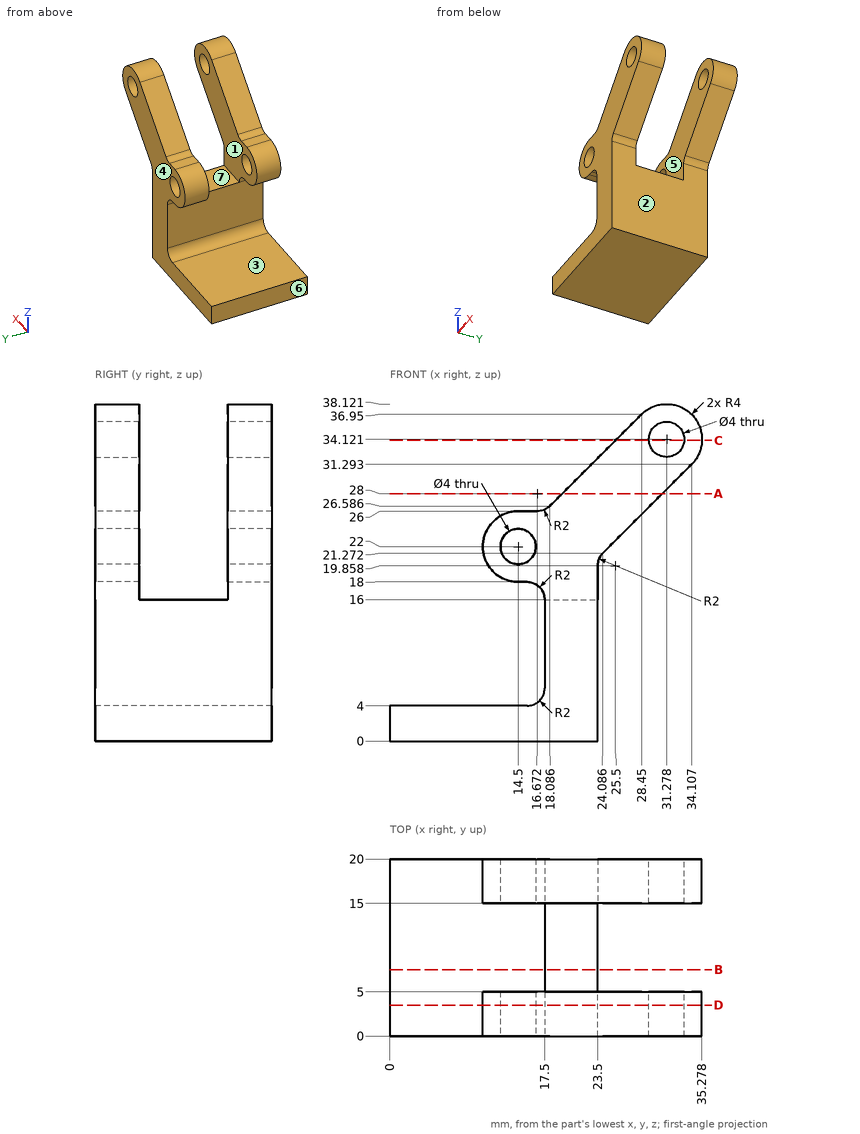
Could you check a few things on this drawing? It's one solid part, dimensions in mm from its lowest x, y, z. A direction names the side the tool comes from. Coordinates: 2 decimals unless noted, no trailing zeros. Order: outer loops, then holes, each group sorted by start corner. A loop starts at its lowest first (then second) coordinate and runs counter-clockwise, first axis right, second up. Notation, with made-up numbers: (61, 54.25) -> (112, 54.25) arc R28 ccw to (112, 90.25) -> close; hole circle Ø1 at (30, 28.25). An arc over 180 degrees is marked (long way). One line per item, written item: value. Start each with the question number.
1) We'd pull the mould along Y, two halves only. Please class the marked faces 4, 5, 6 and 7: +Y half, -Y half, draft (parallel to the pull), parting line (faces both ways), or undercut.
2) Which directions (+Z, -Z, +X, -X, +Y, -Y) give clear straight access to the entire face, cutting with the end or side of a thin tool? Please do the marked faces 1, 2 and 3.
3) Imagine slicing it at B-B on y = 7.5. List the corners of the cut face in (x, z) for me.
4) Imagine slicing it at D-D on y = 3.5. Count the separate pieces of the cut face and the enclosed holes in it, plus the area to 3 significant figures.
5) Imagine slicing it at A-A on z = 28. List the corners of the cut face in (x, y) for me.
6) If I drill on L1, parallel to Z at x = 14.5, y = 3.45; L2, parallel to Y at x = 33.5, z = 32.5; L3, parallel to X at y = 9, z = 11, over which ranges is the centre line in solid material (lowest first)? Write a range as [from, to].
7) I'm going to push flat-ended pins straight in: pin 1 (5 mm diameter, centred on y = 11.5, z = 13, fed in from -X); pin 2 (1.1 mm diameter, centred on x = 15, y = 17.5, fed in from +Z); pin 3 (10 mm diameter, centred on y = 10.5, z = 13.5, fed in from +X). Where does each tip first touch, or does it pass through?
8) Imagine slicing it at C-C on z = 34. List the corners of the cut face in (x, y) for me (1 decimal).
Answer list:
1. face 4: +Y half
1. face 5: undercut
1. face 6: draft
1. face 7: undercut
2. face 1: +Z, +X, -X
2. face 2: -Z, +X, +Y, -Y
2. face 3: -X, +Y, -Y
3. outline: (0, 0) -> (23.5, 0) -> (23.5, 16) -> (17.5, 16) -> (17.5, 6) arc R2 cw to (15.5, 4) -> (0, 4) -> close
4. separate pieces: 1
4. enclosed holes: 2
4. area: 383 mm2
5. outline: (19.5, 0) -> (30.81, 0) -> (30.81, 5) -> (19.5, 5) -> close; (19.5, 15) -> (30.81, 15) -> (30.81, 20) -> (19.5, 20) -> close
6. L1: z = [0, 4], [18, 20], [24, 26]
6. L2: y = [0, 5], [15, 20]
6. L3: x = [17.5, 23.5]
7. pin 1: stops at x = 17.5
7. pin 2: stops at z = 26
7. pin 3: stops at x = 23.5
8. outline: (25.5, 0) -> (29.3, 0) -> (29.3, 5) -> (25.5, 5) -> close; (25.5, 15) -> (29.3, 15) -> (29.3, 20) -> (25.5, 20) -> close; (33.3, 0) -> (35.3, 0) -> (35.3, 5) -> (33.3, 5) -> close; (33.3, 15) -> (35.3, 15) -> (35.3, 20) -> (33.3, 20) -> close
